Check sheet for the drawn part. Datum: minimum x, y, z corner. Units: mm. A direction names the side the tool comes from. Round coordinates to 2 decimals unless told otherwise and drop trailing zeros. Write each loop counter-clockwise with the first axis right and the second up, starting at its lowest first coordinate (ties: lowest second). Pieces come first, ordered by that corner, then holes. Notation, with made-up numbers: (76.25, -18) - (91.25, -18) arc R19 ccw to (91.25, -10) - close; hole circle Ø4 at (55, -7.5). An arc over 180 degrees is marked (long way). Return JSON: item names as keys, results as strings. Group by question number.
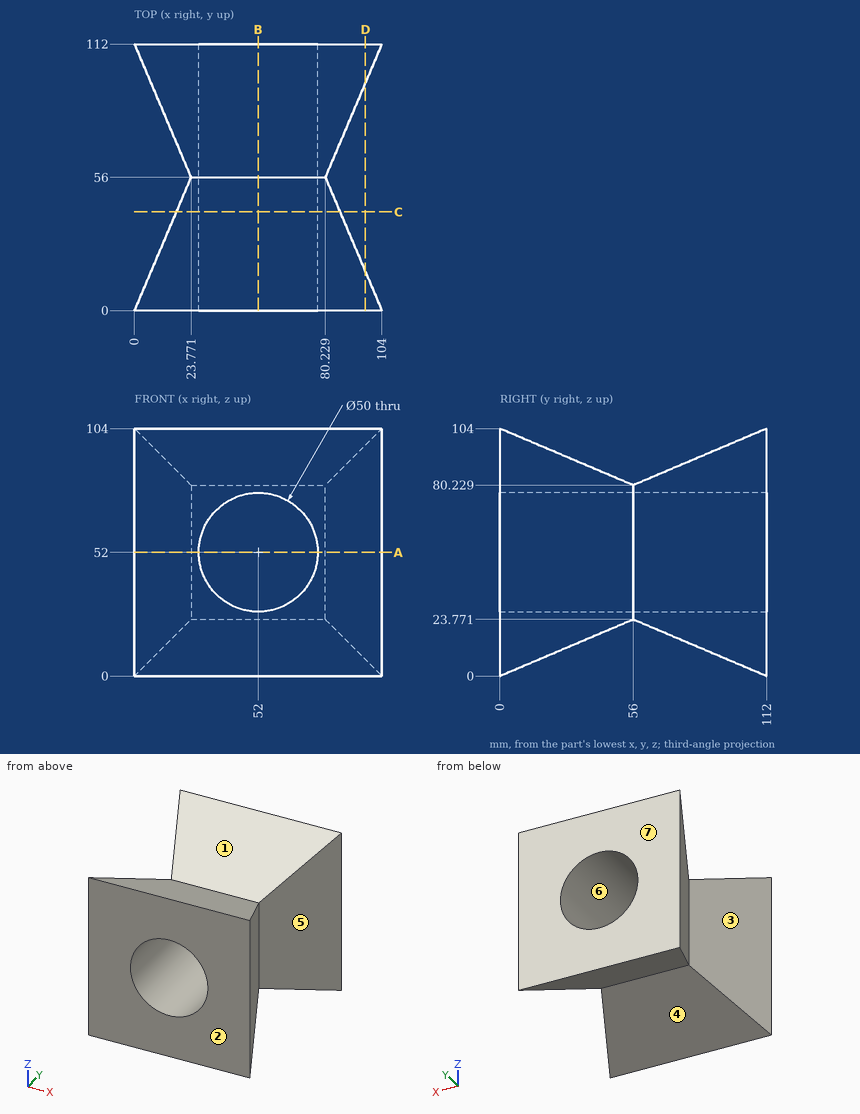
1. Section check C-C (y = 41.5). Enter the section's corners in (x, z) (1 decimal).
2. Section check D-D (x = 97). Enter the section's corners in (y, z).
3. Section check B-B (x = 52). Enter the section's corners in (y, z).
4. Tool access check on the marked faces 1, 2, 3 and 4. Record the directions out of +Z, -Z, +X, -X, +Y, -Y that give a thin tool (end or side, any length) a straight path to the whole face; none if there is none.
5. Depth check by flat-ended pin: pin 1 Ø3 at (y, z) = (86.5, 41.5) entering from +X; pin 2 Ø5 at (x, y) = (19, 96) entering from -Z; pin 3 Ø8 at (x, y) = (52, 42.5) entering from -Z. Enter the tip coordinate at first touch or a pass-through.
6. Material ranges on line 1 along X through (y, z) = (56, 52); line 2 along Y through (x, z) = (98, 89.5) (1 decimal); line 3 along Z through (x, y) = (41.5, 92), recorded low to high.
7. Section check A-A (z = 52). Enter the section's corners in (x, y).
8. Mould release check, pull along Y, two halves, no side actions. Record for the marked faces 5, 6 and 7: pulls with the +Y half, pulls with the -Y half, needs draft (parallel to the pull), parting line crosses it, or undercut.
Result sheet:
{
 "1": {"outline": "(17.6, 17.6) - (86.4, 17.6) - (86.4, 86.4) - (17.6, 86.4) - close; hole circle Ø50 at (52, 52)"},
 "2": {"outline": "(0, 0) - (16.49, 7) - (16.49, 97) - (0, 104) - close; (95.51, 7) - (112, 0) - (112, 104) - (95.51, 97) - close"},
 "3": {"outline": "(0, 0) - (56, 23.77) - (112, 0) - (112, 27) - (0, 27) - close; (0, 77) - (112, 77) - (112, 104) - (56, 80.23) - (0, 104) - close"},
 "4": {"face 1": "+Z, +X, -X", "face 2": "+Z, -Z, +X, -X, -Y", "face 3": "+Z, -Z, -X", "face 4": "-Z, +X, -X"},
 "5": {"pin 1": "stops at x = 93.81", "pin 2": "stops at z = 5.73", "pin 3": "stops at z = 16.34"},
 "6": {"line 1": "x = 23.77 to 27, 77 to 80.23", "line 2": "y = 0 to 14.1, 97.9 to 112", "line 3": "z = 8.49 to 29.31, 74.69 to 95.51"},
 "7": {"outline": "(0, 0) - (27, 0) - (27, 112) - (0, 112) - (23.77, 56) - close; (77, 0) - (104, 0) - (80.23, 56) - (104, 112) - (77, 112) - close"},
 "8": {"face 5": "undercut", "face 6": "needs draft", "face 7": "pulls with the +Y half"}
}
